For this review, take the finished solid that the model builds, in its own axes (mm). A direction names the side the tool comes from. Coordinates: 2 decimals unless noted, no trailing zeros. Write each loop counter-clockwise with the first axis right and the second up, starting at its lowest first coordinate (ties: lowest second). Pieces come first, ordered by that corner, then holes. Notation, with made-up numbers: M 74.5,66 L 86.5,66 A26 ccw 86.5,88 Z; hole C 16.25,9 d4. An arc over 180 degrees is marked long. Return JSON: item names as keys, results as strings.
```python
from build123d import *

# Parameters (mm, degrees)
BOSS_EXTRUDE1_DEPTH = 0.508


with BuildPart() as part:
    # Sketch1 → Boss-Extrude1 (new body)
    with BuildSketch(Plane(origin=(0, 0, 0), x_dir=(1, 0, 0), z_dir=(0, 1, 0))):
        with BuildLine():
            ThreePointArc((26.67, 0), (24.639867132, 10.206167141), (18.858537854, 18.858537854))
            ThreePointArc((18.858537854, 18.858537854), (12.572358569, 18.858537854), (12.572358569, 12.572358569))
            ThreePointArc((12.572358569, 12.572358569), (16.426578088, 6.804111427), (17.78, 0))
            ThreePointArc((17.78, 0), (22.225, -4.445), (26.67, 0))
        make_face()
        with BuildLine():
            ThreePointArc((25.654, 0), (23.701205527, 9.817360774), (18.140117365, 18.140117365))
            ThreePointArc((18.140117365, 18.140117365), (13.290779059, 18.140117365), (13.290779059, 13.290779059))
            ThreePointArc((13.290779059, 13.290779059), (17.365239693, 7.192917795), (18.796, 0))
            ThreePointArc((18.796, 0), (22.225, -3.429), (25.654, 0))
        make_face(mode=Mode.SUBTRACT)
    extrude(amount=BOSS_EXTRUDE1_DEPTH)


solid = part.part
```
1. For faces 4 (the face through (22.15, 0.25, 3.43)), 5 (the face through (17, 0, -7)), list the 3-axis set-ups (+Z, -Z, +X, -X, +Y, -Y) from which the entire face can be reached by the end or side of a thin tool; tool diameter is ignored.
Checks:
{"face 4": "+Y, -Y", "face 5": "+Z, -Z, +X, -X, -Y"}
2. We need section B-B (z = -2.25). State the section outline as (x, y) points, plus the area to 3 significant figures.
Checks:
{"outline": "M 17.64,0 L 18.66,0 L 18.66,0.51 L 17.64,0.51 Z; M 25.56,0 L 26.57,0 L 26.57,0.51 L 25.56,0.51 Z", "area": "1.04 mm2"}
3. Draft analysis for pull direction Z (two halves, no side actions). For faces 1 (the face through (24.696, 0.25, -10.071)), 2 (the face through (17.325, 0.25, -7.288)), 3 (the face through (22.127, 0.25, 4.444)), state which applies: +Z half, -Z half, draft (parallel to the pull), parting line (faces both ways), or undercut.
Checks:
{"face 1": "-Z half", "face 2": "undercut", "face 3": "+Z half"}
4. We need section A-A (y = 0.3). State the section outline as (x, z) points (3 decimals), plus the area to 3 significant figures.
Checks:
{"outline": "M 12.572,-12.572 A4.445 ccw 18.859,-18.859 A26.67 ccw 26.67,0 A4.445 ccw 17.78,0 A17.78 cw Z; hole M 13.291,-13.291 A3.429 ccw 18.14,-18.14 A25.654 ccw 25.654,0 A3.429 ccw 18.796,0 A18.796 cw Z", "area": "60.6 mm2"}
5. Clearance check with a flat-ended pin moving along its axis: pin 1 Ø3 at (x, z) = (17, -9.5) entering from +Y. State where the tip first meets the part, or that it passes through.
Checks:
{"pin 1": "y = 0.51"}
6. We need section C-C (x = 17.25). State the section outline as (y, z) points, plus the area to 3 significant figures.
Checks:
{"outline": "M 0,-19.89 L 0.51,-19.89 L 0.51,-18.78 L 0,-18.78 Z; M 0,-7.47 L 0.51,-7.47 L 0.51,-4.31 L 0,-4.31 Z", "area": "2.16 mm2"}
7. Wall thickness on L1, parallel to X at y = 0.4, z = -15; L2, parallel to X at y = 0.2, z = -13.5; L3, parallel to Z at x = 19.25, y = 0.05: over which ranges is each line inside the solid? List them lowest first. Write a range as from..to.
Checks:
{"L1": "11.33..12.36, 20.81..22.05", "L2": "11.86..13.1, 21.81..23", "L3": "-18.46..-16.96, 1.71..3.3"}
